```python
from build123d import *

# Parameters (mm, degrees)
SKETCH14_W     = 101.6
SKETCH14_H     = 76.2
EXTRUDE5_DEPTH = 19.05
EXTRUDE6_DEPTH = 19.05


with BuildPart() as part:
    # Sketch14 → Extrude5 (new body)
    with BuildSketch(Plane(origin=(0, 0, 0), x_dir=(1, 0, 0), z_dir=(0, 1, 0))):
        with Locations((50.8, 38.1)):
            Rectangle(SKETCH14_W, SKETCH14_H)
    extrude(amount=-EXTRUDE5_DEPTH)

    # Sketch15 → Extrude6 (add)
    with BuildSketch(Plane(origin=(0, 0, 0), x_dir=(1, 0, 0), z_dir=(0, 1, 0))):
        Polygon((101.6, 38.1), (15.359566814, 52.459402124), (15.359566814, 76.2), (101.6, 76.2), align=None)
    extrude(amount=EXTRUDE6_DEPTH)


solid = part.part
```
Verification items for the finished model (mm, model axes). A direction names the side the tool comes from. Give positions to 0.01 mm unless a question says otherwise; leave off trailing zeros. Order: outer loops, then holes, each group sorted by start corner. A loop starts at its lowest first (then second) coordinate and runs counter-clockwise, first axis right, second up. Notation, with made-up numbers: M 73.25,-15 L 86.25,-15 A11 ccw 86.25,-3 Z; hole C -9,50 d5. An arc over 180 degrees is marked long. Answer in a Markdown table with one row per item. Add a question column.
Item 1: Section check A-A, the plane z = -56. Enter the section's corners in (x, y), and give its area (3 significant figures).
Item 2: Section check C-C, the plane x = 49. Enter the section's corners in (y, z).
Item 3: Section check D-D, the plane z = -11.5. Enter the section's corners in (x, y), and give its area (3 significant figures).
Item 4: Gauge pin test, flat ends, axial feed: pin 1 (1 mm diameter, centred on x = 15, z = -41, fed in from +Y); pin 2 (15 mm diameter, centred on y = 8.5, z = -66, fed in from -X). Record the tip position at first contact, or that the pin passes through.
Item 5: Tool access check on faces 1 (the flat face through (50, -19.05, -39)), 2 (the flat face through (15.36, 9, -64)), 3 (the flat face through (59.08, 9.39, -45.18)). Record the directions out of +Z, -Z, +X, -X, +Y, -Y that give a thin tool (end or side, any length) a straight path to the whole face; none if there is none.
Item 6: Section check B-B, the plane y = 6. Enter the section's corners in (x, z).
Item 7: Scan lines: probe 1 along X at (y, z) = (5.5, -64.5); probe 2 along Y at (x, z) = (31.5, -8.5); probe 3 along Z at (x, y) = (37, 12.5). Record each from-to range of solid material in increasing order. Write a range as from..to.
Filled sheet:
| question | item | result |
|---|---|---|
| 1 | outline | M 0,-19.05 L 101.6,-19.05 L 101.6,19.05 L 15.36,19.05 L 15.36,0 L 0,0 Z |
| 1 | area | 3,580 mm^2 |
| 2 | outline | M -19.05,-76.2 L 19.05,-76.2 L 19.05,-46.86 L 0,-46.86 L 0,0 L -19.05,0 Z |
| 3 | outline | M 0,-19.05 L 101.6,-19.05 L 101.6,0 L 0,0 Z |
| 3 | area | 1,940 mm^2 |
| 4 | pin 1 | stops at y = 0 |
| 4 | pin 2 | stops at x = 15.36 |
| 5 | face 1 | +Z, -Z, +X, -X, -Y |
| 5 | face 2 | +Z, -Z, -X, +Y |
| 5 | face 3 | +Z, -X, +Y |
| 6 | outline | M 15.36,-76.2 L 101.6,-76.2 L 101.6,-38.1 L 15.36,-52.46 Z |
| 7 | probe 1 | x = 15.36..101.6 |
| 7 | probe 2 | y = -19.05..0 |
| 7 | probe 3 | z = -76.2..-48.86 |
